The model under review builds one solid part; all positions refer to its coordinate system, in mm. Face numbers are marked on the shaded views. A direction names the side the tool comes from. Round coordinates to 2 decimals unless told otherwise and drop trailing zeros. Write each loop counter-clockwise with the first axis right and the second up, starting at its lowest first coordinate (ties: lowest second). Pieces come first, ordered by that corner, then holes. Notation, with made-up numbers: (13.5, 15.5) - (69.5, 15.5) arc R29 ccw to (69.5, 40.5) - close; hole circle Ø7 at (8, 59.5). An arc over 180 degrees is marked (long way). One line per question, with ' | ' between items. Start each with the question number.
```python
from build123d import *

# Parameters (mm, degrees)
SKETCH_1_R               = 2.5
EXTRUDE_654_DEPTH        = 12
CHAMFER_1_SIZE           = 0.8
CUT_EXTRUDE_1_DEPTH      = 14.649908425
CUT_EXTRUDE_1_DEPTH_BACK = 14.649908425
SKETCH_4_W               = 1.2
SKETCH_4_H               = 1.35


with BuildPart() as part:
    # Эскиз1 → Extrude 654 (new body)
    with BuildSketch(Plane(origin=(0, 0, 0), x_dir=(0, 0, -1), z_dir=(1, 0, 0))):
        Circle(SKETCH_1_R)
    extrude(amount=EXTRUDE_654_DEPTH)

    # Фаска1
    chamfer_1_edges = [part.edges().sort_by_distance(p)[0] for p in [
        (12, 0, 2.5),
    ]]
    chamfer(chamfer_1_edges, length=CHAMFER_1_SIZE)

    # Эскиз2 → Бобышка-Повернуть1 (revolve)
    with BuildSketch(Plane.XY, mode=Mode.PRIVATE) as revolve_1_sk:
        Polygon((0, 4.6), (0.4, 4.6), (2.5, 2.5), (2.5, 0), (0, 0), align=None)
    revolve(revolve_1_sk.sketch.rotate(Axis((0, 0, 0), (1, 0, 0)), 90), axis=Axis((0, 0, 0), (1, 0, 0)))

    # Эскиз4 → Вырез-Вытянуть1 (cut, two sides: drawn at the far end of the back side and taken through both)
    with BuildSketch(Plane.XY.offset(-CUT_EXTRUDE_1_DEPTH_BACK)):
        with Locations((0.6, 0)):
            Rectangle(SKETCH_4_W, SKETCH_4_H)
    extrude(amount=CUT_EXTRUDE_1_DEPTH + CUT_EXTRUDE_1_DEPTH_BACK, mode=Mode.SUBTRACT)


solid = part.part
```
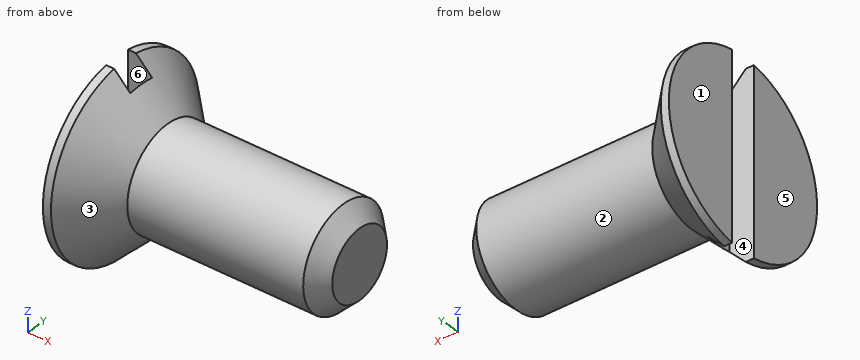
1. Machinability: for the marked faces 1 and 2, which of the approach directions +Z, -Z, +X, -X, +Y, -Y give a long, thin tool a straight path to every point of the face, cutting with its end or side? Answer none if there is none.
2. Add section B-B, the plane z = 0. Write out the cut boundary in (x, y) (3 decimals), then the cut area to 3 significant figures.
3. Clearance check with flat-ended pins moving along their axes: P1, Ø1, axis at x = 6, y = 0.5, coming from the +Z side; P2, Ø3, axis at x = 6, z = -2.5, coming from the +Y side; P3, Ø1, axis at x = 1, z = -1, coming from the -Y side. State where each tip first meets the part, or that it passes through.
4. Wall thickness on line 1 along X through (y, z) = (0, 1.5); line 2 along Y through (x, z) = (2, -0.75); line 3 along X through (y, z) = (-1.5, -3.75): over which ranges is each line inside the solid? List them lowest first. Write a range as [from, to].
5. Add section A-A, the plane y = 0. Write out the cut boundary in (x, z).
6. Add section C-C, the plane x = 3.25. Write out the cut boundary in (y, z), then the cut area to 3 significant figures.
7. The part is to be moulded in two halves that separate along Y. For the marked faces 3, 4, 5 and 6, say which applies: pulls with the +Y half, pulls with the -Y half, needs draft (parallel to the pull), parting line crosses it, or undercut.
Geometry check:
1) face 1: +Z, -Z, -X, +Y, -Y | face 2: +X
2) outline: (0, -4.6) - (0.4, -4.6) - (2.5, -2.5) - (11.2, -2.5) - (12, -1.7) - (12, 1.7) - (11.2, 2.5) - (2.5, 2.5) - (0.4, 4.6) - (0, 4.6) - (0, 0.675) - (1.2, 0.675) - (1.2, -0.675) - (0, -0.675) - close | area: 63.8 mm2
3) P1: stops at z = 2.5 | P2: stops at y = 2.29 | P3: stops at y = -4.4
4) line 1: x = [1.2, 12] | line 2: y = [-2.9, 2.9] | line 3: x = [0, 0.96]
5) outline: (1.2, -3.8) - (2.5, -2.5) - (11.2, -2.5) - (12, -1.7) - (12, 1.7) - (11.2, 2.5) - (2.5, 2.5) - (1.2, 3.8) - close
6) outline: circle Ø5 at (0, 0) | area: 19.6 mm2
7) face 3: parting line crosses it | face 4: undercut | face 5: needs draft | face 6: undercut
